Part print with two shaded views. Sizes in mm from the minimum x, y, z corner. A direction names the side the tool comes from. Give positions to 0.01 mm unless a question says otherwise; leave off trailing zeros. Order: outer loops, then holes, each group sorted by start corner. A loop starts at its lowest first (then second) coordinate and runs counter-clockwise, first axis right, second up. Notation, with made-up numbers: M -14.5,79.5 L -10.5,79.5 A20 ccw -10.5,92.5 Z; hole C -5,54.5 d8. An arc over 180 degrees is marked long. Return JSON: item names as keys, results as strings.
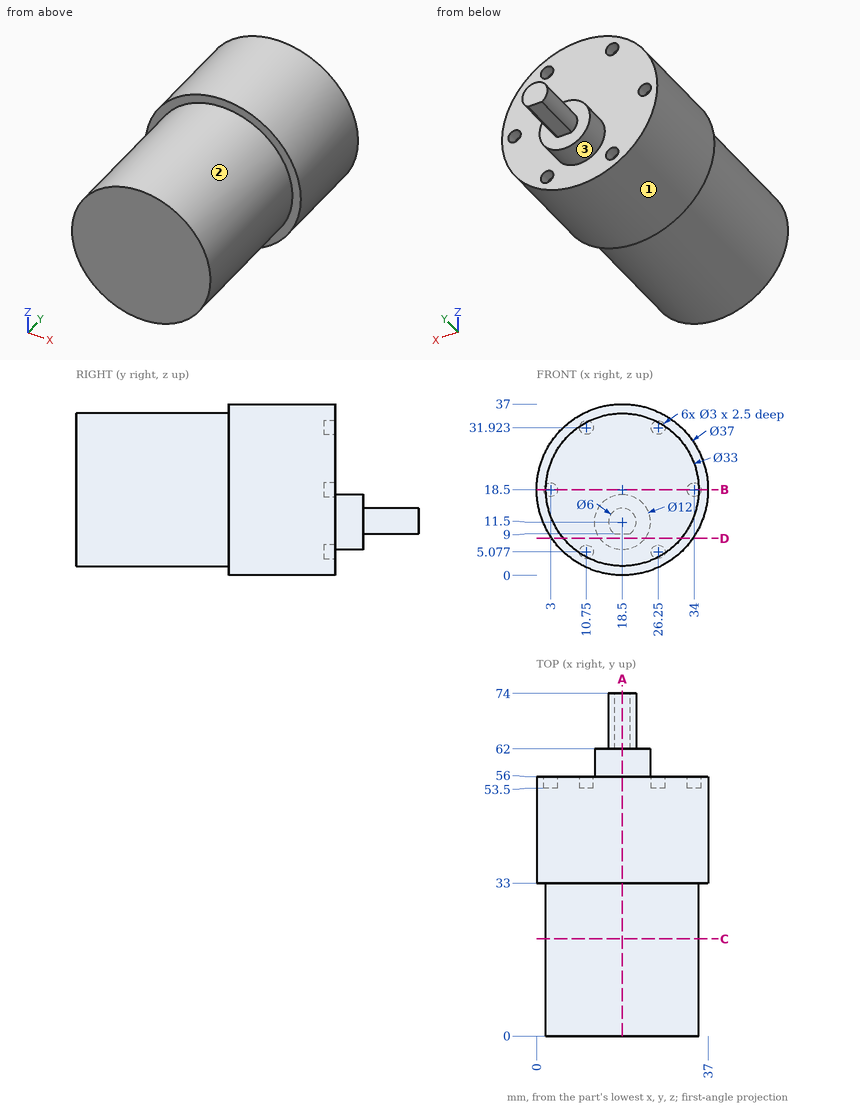
Q1. Band-saw the part on C-C (y = 21). Give the cut face in (x, z).
Established:
{"outline": "C 18.5,18.5 d33"}
Q2. Probe line 1 along X through (y, z) = (54, 18) (1 decimal); line 2 along Y through (x, z) = (17.5, 18); line 3 along X through (y, z) = (5.5, 18). List the from-to ranges inside material, lowest first.
Established:
{"line 1": "x = 0 to 1.6, 4.4 to 32.6, 35.4 to 37", "line 2": "y = 0 to 56", "line 3": "x = 2.01 to 34.99"}
Q3. Band-saw the part on B-B (z = 18.5). Give the cut face in (x, y), then the cut area to 4 significant figures.
Established:
{"outline": "M 0,33 L 2,33 L 2,0 L 35,0 L 35,33 L 37,33 L 37,56 L 35.5,56 L 35.5,53.5 L 32.5,53.5 L 32.5,56 L 4.5,56 L 4.5,53.5 L 1.5,53.5 L 1.5,56 L 0,56 Z", "area": "1,925 mm²"}
Q4. Band-saw the part on D-D (z = 8). Give the cut face in (x, y).
Established:
{"outline": "M 3.27,33 L 5.77,33 L 5.77,0 L 31.23,0 L 31.23,33 L 33.73,33 L 33.73,56 L 23.37,56 L 23.37,62 L 13.63,62 L 13.63,56 L 3.27,56 Z"}
Q5. Pin check, flat tips, straight feed: pin 1 (4 mm diameter, centred on x = 22.5, z = 6.5, fed in from -Y); pin 2 (2.5 mm diameter, centred on x = 26, z = 5.5, fed in from +Y); pin 3 (8 mm diameter, centred on y = 12, z = 6.5, fed in from +X); pin 4 (1.5 mm diameter, centred on x = 31, y = 39.5, fed in from -Z). Stop position of each tip, or through.
Established:
{"pin 1": "stops at y = 0", "pin 2": "stops at y = 56", "pin 3": "stops at x = 32.93", "pin 4": "stops at z = 4.21"}
Q6. 3-axis set-ups, long thin cutter, end or side, ignore diameter. For the marked faces 1, 2 and 3: which of +Z, -Z, +X, -X, +Y, -Y reach the whole face in a straight line?
Established:
{"face 1": "+Y, -Y", "face 2": "-Y", "face 3": "+Y"}
Q7. Band-saw the part on A-A (x = 18.5). Give the cut face in (y, z).
Established:
{"outline": "M 0,2 L 33,2 L 33,0 L 56,0 L 56,5.5 L 62,5.5 L 62,9 L 74,9 L 74,14.5 L 62,14.5 L 62,17.5 L 56,17.5 L 56,37 L 33,37 L 33,35 L 0,35 Z"}
